Build history of the part. All positions in model axes, mm. A direction names the side the tool comes from. Round coordinates to 2 decimals unless told otherwise and drop trailing zeros. Order: outer loops, then holes, each group sorted by start corner. A loop starts at its lowest first (then second) coordinate and runs counter-clockwise, first axis right, second up. Notation, with made-up numbers: (-11, 56.25) -> (-7, 56.25) arc R30 cw to (-7, 82.25) -> close; hole circle Ø5 at (-25.75, 52). An arc over 180 degrees is marked (long way). Answer as a JSON object with one key per item and string values.
from build123d import *

# Parameters (mm, degrees)
F0_W      = 69.85
F0_H      = 38.1
F1_DEPTH  = 25.4
F2_W      = 44.45
F2_H      = 25.4
F3_DEPTH  = 25.401
F5_DEPTH  = 25.401
F7_DEPTH  = 25.401
F9_DEPTH  = 12.701
F10_W     = 22.1024058417
F10_H     = 12.7
F11_DEPTH = 25.4
F13_DEPTH = 12.701


with BuildPart() as f1:
    # F0 (on Front) → F1 (new body)
    with BuildSketch(Plane.XZ):
        with Locations((-0.1225941583, 19.05)):
            Rectangle(F0_W, F0_H)
    extrude(amount=F1_DEPTH)

    # F2 (on face) → F3 (cut, through all)
    with BuildSketch(Plane.XZ.offset(25.4)):
        with Locations((12.5774058417, 25.4)):
            Rectangle(F2_W, F2_H)
    extrude(amount=-F3_DEPTH, mode=Mode.SUBTRACT)

    # F4 (on face) → F5 (cut, through all)
    with BuildSketch(Plane.XZ.offset(25.4)):
        with BuildLine():
            Line((-9.6475941583, 38.1), (-22.3475941583, 38.1))
            ThreePointArc((-22.3475941583, 38.1), (-13.3673380372, 34.3802561211), (-9.6475941583, 25.4))
            Line((-9.6475941583, 25.4), (-9.6475941583, 38.1))
        make_face()
        with BuildLine():
            Line((-22.3475941583, 38.1), (-35.0475941583, 38.1))
            Line((-35.0475941583, 38.1), (-35.0475941583, 25.4))
            ThreePointArc((-35.0475941583, 25.4), (-31.3278502794, 34.3802561211), (-22.3475941583, 38.1))
        make_face()
    extrude(amount=-F5_DEPTH, mode=Mode.SUBTRACT)

    # F6 (on face) → F7 (cut, through all)
    with BuildSketch(Plane.XZ.offset(25.4)):
        with BuildLine():
            ThreePointArc((-22.3475941583, 31.75), (-26.8377222188, 29.8901280605), (-28.6975941583, 25.4))
            Line((-28.6975941583, 25.4), (-22.3475941583, 25.4))
            Line((-22.3475941583, 25.4), (-22.3475941583, 31.75))
        make_face()
        with BuildLine():
            Line((-22.3475941583, 31.75), (-22.3475941583, 25.4))
            Line((-22.3475941583, 25.4), (-15.9975941583, 25.4))
            ThreePointArc((-15.9975941583, 25.4), (-17.8574660977, 29.8901280605), (-22.3475941583, 31.75))
        make_face()
        with BuildLine():
            Line((-15.9975941583, 25.4), (-22.3475941583, 25.4))
            Line((-22.3475941583, 25.4), (-22.3475941583, 19.05))
            ThreePointArc((-22.3475941583, 19.05), (-17.8574660977, 20.9098719395), (-15.9975941583, 25.4))
        make_face()
        with BuildLine():
            Line((-22.3475941583, 25.4), (-28.6975941583, 25.4))
            ThreePointArc((-28.6975941583, 25.4), (-26.8377222188, 20.9098719395), (-22.3475941583, 19.05))
            Line((-22.3475941583, 19.05), (-22.3475941583, 25.4))
        make_face()
    extrude(amount=-F7_DEPTH, mode=Mode.SUBTRACT)

    # F8 (on face) → F9 (cut, through all)
    with BuildSketch(Plane.XY.offset(12.7)):
        with BuildLine():
            Line((28.4524058417, 0), (22.1024058417, 0))
            ThreePointArc((22.1024058417, 0), (31.0826619628, -3.7197438789), (34.8024058417, -12.7))
            Line((34.8024058417, -12.7), (34.8024058417, 0))
            Line((34.8024058417, 0), (28.4524058417, 0))
        make_face()
        with BuildLine():
            ThreePointArc((34.8024058417, -12.7), (31.0826619628, -21.6802561211), (22.1024058417, -25.4))
            Line((22.1024058417, -25.4), (28.4524058417, -25.4))
            Line((28.4524058417, -25.4), (34.8024058417, -25.4))
            Line((34.8024058417, -25.4), (34.8024058417, -12.7))
        make_face()
    extrude(amount=-F9_DEPTH, mode=Mode.SUBTRACT)

    # F10 (on face) → F11 (cut)
    with BuildSketch(Plane.XY.offset(12.7)):
        with Locations((11.0512029209, -12.7)):
            Rectangle(F10_W, F10_H)
    extrude(amount=-F11_DEPTH, mode=Mode.SUBTRACT)

    # F12 (on face) → F13 (cut, through all)
    with BuildSketch(Plane.XY.offset(12.7)):
        with BuildLine():
            ThreePointArc((0, -6.35), (-6.35, -12.7), (0, -19.05))
            Line((0, -19.05), (0, -6.35))
        make_face()
        with BuildLine():
            Line((22.1024058417, -6.35), (22.1024058417, -19.05))
            ThreePointArc((22.1024058417, -19.05), (28.4524058417, -12.7), (22.1024058417, -6.35))
        make_face()
    extrude(amount=-F13_DEPTH, mode=Mode.SUBTRACT)


solid = f1.part
1) Cut at D-D, the plane z = 22. Give the cut face in (x, y).
Checked values:
{"outline": "(-35.05, -25.4) -> (-27.71, -25.4) -> (-27.71, 0) -> (-35.05, 0) -> close; (-16.98, -25.4) -> (-9.65, -25.4) -> (-9.65, 0) -> (-16.98, 0) -> close"}
2) Which spindle directions (+Z, -Z, +X, -X, +Y, -Y) get a long thin tool onto all of the face, cutting with end or side? Do faces 4 (the face through (-9.648, -13, 19)), 5 (the face through (-8, -13, 0)), 6 (the face through (11, -19.05, 6)). Say none if no direction does.
Checked values:
{"face 4": "+Z, +X, +Y, -Y", "face 5": "-Z, +X, -X, +Y, -Y", "face 6": "+Z, -Z"}
3) Flat gauge pins, fed straight in: pin 1 Ø5 at (y, z) = (-15.5, 15) entering from +X; pin 2 Ø1 at (x, z) = (-16.5, 13) entering from +Y; pin 3 Ø4 at (y, z) = (-16.5, 18.5) entering from +X; pin 4 Ø6 at (y, z) = (-12.5, 31) entering from +X. Where does each tip first touch, or does it go through?
Checked values:
{"pin 1": "stops at x = 34.67", "pin 2": "stops at y = 0", "pin 3": "stops at x = -9.65", "pin 4": "stops at x = -9.92"}
4) Cut at A-A, the plane x = 20.5. Give the cut face in (y, z), plus the area to 3 significant figures.
Checked values:
{"outline": "(-25.4, 0) -> (-19.05, 0) -> (-19.05, 12.7) -> (-25.4, 12.7) -> close; (-6.35, 0) -> (0, 0) -> (0, 12.7) -> (-6.35, 12.7) -> close", "area": "161 mm²"}
5) Pull direction Y, two halves, no side cores. Call faces 1 (the face through (11, -6.35, 6)), 2 (the face through (-13, 0, 15)), 3 (the face through (-35.048, -13, 13)): pulls with the +Y half, pulls with the -Y half, needs draft (parallel to the pull), parting line crosses it, or undercut.
Checked values:
{"face 1": "undercut", "face 2": "pulls with the +Y half", "face 3": "needs draft"}
6) Cut at C-C, the plane z = 7.5. Give the cut face in (x, y), plus the area to 3 significant figures.
Checked values:
{"outline": "(-35.05, -25.4) -> (22.1, -25.4) arc R12.7 ccw to (22.1, 0) -> (-35.05, 0) -> close; hole (0, -19.05) -> (22.1, -19.05) arc R6.35 ccw to (22.1, -6.35) -> (0, -6.35) arc R6.35 ccw to start", "area": "1,300 mm²"}
7) Cut at B-B, the plane y = -18.25. Give the cut face in (x, z).
Checked values:
{"outline": "(-35.05, 0) -> (-3.09, 0) -> (-3.09, 12.7) -> (-9.65, 12.7) -> (-9.65, 25.4) arc R12.7 ccw to (-35.05, 25.4) -> close; (25.19, 0) -> (33.53, 0) -> (33.53, 12.7) -> (25.19, 12.7) -> close; hole circle Ø12.7 at (-22.35, 25.4)"}
8) Probe L1, parallel to Y at x = 0.5, z = 10.5; L2, parallel to X at y = -20.5, z = 16. List the from-to ranges inside material, lowest first. Write a range as from..to.
Checked values:
{"L1": "y = -25.4..-19.05, -6.35..0", "L2": "x = -35.05..-9.65"}
